```python
from build123d import *

# Parameters (mm, degrees)
F0_R     = 5
F1_DEPTH = 7
F0_R_2   = 8
F2_DEPTH = 1.2
F3_R     = 0.5


with BuildPart() as f1:
    # F0 (on Top) → F1 (new body)
    with BuildSketch(Plane.XY):
        Circle(F0_R)
        with BuildLine():
            ThreePointArc((1.05, 1.4), (1.5652475842, 0.7826237921), (1.75, 0))
            ThreePointArc((1.75, 0), (1.5652475842, -0.7826237921), (1.05, -1.4))
            ThreePointArc((1.05, -1.4), (-0.7826237921, -1.5652475842), (-1.75, 0))
            ThreePointArc((-1.75, 0), (-0.7826237921, 1.5652475842), (1.05, 1.4))
        make_face(mode=Mode.SUBTRACT)
        with BuildLine():
            ThreePointArc((1.05, -1.4), (1.5652475842, -0.7826237921), (1.75, 0))
            ThreePointArc((1.75, 0), (1.5652475842, 0.7826237921), (1.05, 1.4))
            Line((1.05, 1.4), (1.05, 0))
            Line((1.05, 0), (1.05, -1.4))
        make_face()
    extrude(amount=F1_DEPTH)

    # F0 (on Top) → F2 (join)
    with BuildSketch(Plane.XY):
        Circle(F0_R_2)
        Circle(F0_R, mode=Mode.SUBTRACT)
    extrude(amount=F2_DEPTH)

    # F3
    f3_edges = [f1.edges().sort_by_distance(p)[0] for p in [
        (-8, 0, 1.2),
    ]]
    fillet(f3_edges, radius=F3_R)


solid = f1.part
```
Verification items for the finished model (mm, model axes). Give positions to 0.01 mm unless a question says otherwise; leave off trailing zeros. Order: outer loops, then holes, each group sorted by start corner. A loop starts at its lowest first (then second) coordinate and runs counter-clockwise, first axis right, second up. Notation, with made-up numbers: M -15,32.5 L 2,32.5 A22 ccw 2,45.5 Z; hole C 77.25,-12.75 d1. An arc over 180 degrees is marked long. Return JSON: item names as keys, results as strings. Group by question number.
1) Scan lines: line 1 (Z direction, x = 2.75, y = 7); line 2 (X direction, y = -1.5, z = 1.5); line 3 (Y direction, x = -1, z = 3). Record each from-to range of solid material in increasing order.
2) Mould release check, pull along Y, two halves, no side actions. Record for faces 1 (the face through (5, -2, 1.2)), 2 (the face through (1.05, 0, 3)), 3 (the face through (-1.08, -4.88, 4.06)): pulls with the +Y half, pulls with the -Y half, needs draft (parallel to the pull), parting line crosses it, or undercut.
3) Section check B-B on z = 1.75. Record the cut outline in (x, y), and give its area (3 significant figures).
4) Section check A-A on x = 0. Record the cut outline in (y, z), and give its area (3 significant figures).
5) Go/stop test with flat-tipped pins: pin 1 Ø1 at (x, z) = (-3.5, 5) entering from -Y; pin 2 Ø2 at (x, z) = (5, 4.5) entering from -Y; pin 3 Ø0.8 at (y, z) = (0.5, 4) entering from -X. Record where each tip stops, or that it passes through.
Answer block:
{
 "1": {"line 1": "z = 0 to 1.2", "line 2": "x = -4.77 to -0.9, 0.9 to 4.77", "line 3": "y = -4.9 to -1.44, 1.44 to 4.9"},
 "2": {"face 1": "needs draft", "face 2": "undercut", "face 3": "parting line crosses it"},
 "3": {"outline": "C 0,0 d10; hole M 1.05,-1.4 L 1.05,1.4 A1.75 ccw long Z", "area": "70.3 mm^2"},
 "4": {"outline": "M -8,0 L -1.75,0 L -1.75,7 L -5,7 L -5,1.2 L -7.5,1.2 A0.5 ccw -8,0.7 Z; M 1.75,0 L 8,0 L 8,0.7 A0.5 ccw 7.5,1.2 L 5,1.2 L 5,7 L 1.75,7 Z", "area": "52.6 mm^2"},
 "5": {"pin 1": "stops at y = -4", "pin 2": "stops at y = -3", "pin 3": "stops at x = -5"}
}
